```python
from build123d import *

# Parameters (mm, degrees)
F1_DEPTH = 6
F2_D     = 12.5
F3_D     = 5
F4_D     = 5
F5_D     = 5
F6_R     = 5
F7_D     = 8
F7_DEPTH = 20
F7_TIP   = 2.4034424761


with BuildPart() as f1:
    # F0 (on Front) → F1 (new body)
    with BuildSketch(Plane.XZ):
        Polygon((0, 27), (0, -27), (13, -27), (40, -27), (40, 38), (26, 38), (26, 73), (0, 73), align=None)
    extrude(amount=F1_DEPTH)

    # F2 (through all)
    with Locations(Plane(origin=(0, 0, 0), x_dir=(1, 0, 0), z_dir=(0, 1, 0))):
        with Locations((13, 7)):
            Hole(F2_D / 2)

    # F3 (through all)
    with Locations(Plane(origin=(0, 0, 0), x_dir=(1, 0, 0), z_dir=(0, 1, 0))):
        with Locations((34, 21), (34, -32)):
            Hole(F3_D / 2)

    # F4 (through all)
    with Locations(Plane(origin=(0, 0, 0), x_dir=(1, 0, 0), z_dir=(0, 1, 0))):
        with Locations((5, -32), (21, -32)):
            Hole(F4_D / 2)

    # F5 (through all)
    with Locations(Plane(origin=(0, 0, 0), x_dir=(1, 0, 0), z_dir=(0, 1, 0))):
        with Locations((5, -68), (21, -68)):
            Hole(F5_D / 2)

    # F6
    f6_edges = [f1.edges().sort_by_distance(p)[0] for p in [
        (0, -3, 73),
        (26, -3, 73),
        (26, -3, 38),
        (40, -3, 38),
        (40, -3, -27),
        (0, -3, -27),
    ]]
    fillet(f6_edges, radius=F6_R)

    # F7
    with Locations(Plane(origin=(0, 0, 0), x_dir=(1, 0, 0), z_dir=(0, 1, 0))):
        with Locations((13, -55.5)):
            Hole(F7_D / 2, depth=F7_DEPTH)
            with Locations((0, 0, -(F7_DEPTH + F7_TIP / 2))):  # 118° drill point
                Cone(0, F7_D / 2, F7_TIP, mode=Mode.SUBTRACT)


solid = f1.part
```
Build history of the part. All positions in model axes, mm. A direction names the side the tool comes from. Round coordinates to 2 decimals unless told otherwise and drop trailing zeros. Write each loop counter-clockwise with the first axis right and the second up, starting at its lowest first coordinate (ties: lowest second). Pieces come first, ordered by that corner, then holes. Notation, with made-up numbers: (74, 56.5) - (106, 56.5) arc R18 cw to (106, 70.5) - close; hole circle Ø7 at (-15, 86). An arc over 180 degrees is marked (long way). Write each question's results on one line, items separated by ' | '. Start each with the question number.
Item 1: Saw through at D-D (z = 55.5). Write the cut outline in (x, y).
Item 2: Which spindle directions (+Z, -Z, +X, -X, +Y, -Y) get a long thin tool onto all of the face, cutting with end or side? Do faces 5 (the face through (32.66, -3.04, -23.11)), 6 (the face through (26, -3, 55)). Say none if no direction does.
Item 3: Mould opens along Z. For faces 1 (the face through (33, -3, 38)), 2 (the face through (2, -3, -26)), 3 (the face through (0, -3, 24)), 4 (the face through (13.867, -3.042, 59.405)) say: pulls with the +Z half, pulls with the -Z half, needs draft (parallel to the pull), parting line crosses it, or undercut.
Item 4: Drop flat-ended pins along their axis: P1, Ø6.5, axis at x = 34, z = 32, coming from the +Y side; P2, Ø3, axis at x = 25.5, y = -2, coming from the +Z side; P3, Ø3, axis at y = -3, z = 54.5, coming from the +X side. Give the stop position or say it passes through.
Item 5: Saw through at C-C (y = -3.55). State how many separate pieces and enclosed holes the cut face has, and give its area (3 significant figures).
Item 6: Wall check: L1, parallel to X at y = -1.3, z = 32; L2, parallel to Z at x = 21, y = -3.55; L3, parallel to X at y = -1.9, z = 68. Give the ranges that are in metal, low to high. Write a range as [from, to].
Item 7: Saw through at A-A (x = 13). Write the cut outline in (y, z), and give its area (3 significant figures).
Item 8: Saw through at B-B (z = -7). Write the cut outline in (x, y).
Results are:
1) outline: (0, -6) - (9, -6) - (9, 0) - (0, 0) - close; (17, -6) - (26, -6) - (26, 0) - (17, 0) - close
2) face 5: +Y, -Y | face 6: +Z, +X, +Y, -Y
3) face 1: pulls with the +Z half | face 2: pulls with the -Z half | face 3: needs draft | face 4: undercut
4) P1: stops at y = 0 | P2: stops at z = 72 | P3: stops at x = 26
5) separate pieces: 1 | enclosed holes: 8 | area: 3,200 mm²
6) L1: x = [0, 2.5], [7.5, 18.5], [23.5, 31.5], [36.5, 40] | L2: z = [-27, 29.5], [34.5, 65.5], [70.5, 73] | L3: x = [0, 2.5], [7.5, 18.5], [23.5, 26]
7) outline: (-6, -27) - (0, -27) - (0, -13.25) - (-6, -13.25) - close; (-6, -0.75) - (0, -0.75) - (0, 51.5) - (-6, 51.5) - close; (-6, 59.5) - (0, 59.5) - (0, 73) - (-6, 73) - close | area: 477 mm²
8) outline: (0, -6) - (6.75, -6) - (6.75, 0) - (0, 0) - close; (19.25, -6) - (40, -6) - (40, 0) - (19.25, 0) - close
